Autodesk Inventor part; units mm, degrees
ref_plane "YZ Plane" through (0, 0, 0) normal (1, 0, 0) x (0, 1, 0)
ref_plane "XZ Plane" through (0, 0, 0) normal (0, 1, 0) x (-1, 0, 0)
ref_plane "XY Plane" through (0, 0, 0) normal (0, 0, 1) x (1, 0, 0)
sketch "Sketch1" plane through (0, 0, 0) normal (1, 0, 0) x (0, 1, 0)
  line L0 (0, 0) -> (3.175, 0)
  line L1 (3.175, -12.7) -> (0, -12.7)
  line L2 (0, -12.7) -> (0, 0)
  line L3 (3.175, 0) -> (28.575, 0)
  line L4 (3.175, -12.7) -> (28.575, -12.7)
  line L5 (12.065, -4.1275) -> (28.575, 0)
  line L6 (12.065, -8.5725) -> (28.575, -12.7)
  line L7 (12.065, -4.1275) -> (3.175, -4.1275)
  line L8 (12.065, -8.5725) -> (3.175, -8.5725)
  line L9 (3.175, -4.1275) -> (2.54, -4.1275)
  line L10 (2.54, -4.1275) -> (2.54, -8.5725)
  line L11 (2.54, -8.5725) -> (3.175, -8.5725)
  dimension "d0" = 3.175
  dimension "d1" = 12.7
  dimension "d2" = 25.4
  dimension "d3" = 0.635
extrude "Extrusion1" add sketch "Sketch1" along normal blind 88.9
sketch "Sketch2" plane through (0, 0, 0) normal (0, 0, 1) x (1, 0, 0)
  line L0 (70.7723, 45.5937) -> (70.7723, 36.3388)
  line L1 (0, 12.065) -> (88.9, 12.065)
  line L2 (70.7723, 36.3388) -> (70.7723, 45.5937)
  line L3 (70.7723, 45.5937) -> (88.9, 45.5937)
  line L4 (88.9, 45.5937) -> (70.7723, 45.5937)
  line L5 (70.7723, 45.5937) -> (79.5643, 35.1158)
  line L6 (88.9, 12.065) -> (88.9, 28.575)
  line L7 (88.9, 28.575) -> (57.2257, 28.575)
  line L8 (0, 28.575) -> (88.9, 28.575)
  line L9 (88.9, 0) -> (76.2, 0)
  line L10 (0, 0) -> (88.9, 0)
  line L11 (76.2, 0) -> (52.2227, 28.575)
  line L12 (52.2227, 28.575) -> (52.2227, 24.9497)
  line L13 (0, 28.575) -> (0, 0)
  line L14 (0, 0) -> (88.9, 0)
  line L15 (88.9, 28.575) -> (88.9, 0)
  line L16 (0, 28.575) -> (88.9, 28.575)
  dimension "d6" = 40
  dimension "d8" = 12.7
  dimension "d9" = 40
extrude "Extrusion2" add sketch "Sketch2" against normal blind 12.7 contours L11 L8 L7 L6 L1 | L1 L15 L9 L11
sketch "Sketch3" plane through (0, 0, 0) normal (0, 0, 1) x (1, 0, 0)
  line L0 (0, 28.575) -> (52.2227, 28.575)
  line L1 (52.2227, 28.575) -> (58.5727, 28.575)
  line L2 (52.2227, 28.575) -> (88.9, 28.575)
  line L3 (52.2227, 28.575) -> (66.0763, 12.065)
  line L4 (58.5727, 28.575) -> (89.629, -8.4365)
  line L5 (58.5727, 28.575) -> (106.8878, 28.575) construction
  line L6 (89.629, -8.4365) -> (99.364, 12.7806)
  line L7 (99.364, 12.7806) -> (87.0878, 39.7231)
  line L8 (87.0878, 39.7231) -> (61.7749, 33.0961)
  line L9 (61.7749, 33.0961) -> (58.5727, 28.575)
  point P0 (0, 0)
  dimension "d12" = 6.35
  dimension "d13" = 50
extrude "Extrusion3" cut sketch "Sketch3" against normal blind 12.7
properties part number "edge holder tip"
Geometry: final body of the model. Coordinates: model frame, mm. A direction names the side the tool comes from. Give positions to 0.01 mm unless a question says otherwise; leave off trailing zeros. Write each loop counter-clockwise with the first axis right and the second up, starting at its lowest first coordinate (ties: lowest second). Pieces come first, ordered by that corner, then holes.
(1) Cut plane B-B, the plane y = 23. Return loops of the section in (x, z), then the cut area to 3 significant figures.
(2) Mould query, pull axis Z, two halves, no side actions, for faces 1 (the flat face through (37, 7, -4.128)), 2 (the flat face through (37, 7, -8.572)), 3 (the flat face through (32, 14, 0)), 4 (the flat face through (0, 11, -3)). Classes: released by +Z, released by -Z, zero draft, split by the parting line, or undercut.
(3) Cut plane A-A, the plane x = 26.5. Return loops of the section in (y, z) (1 decimal), then the cut area to 3 significant figures.
(4) First-contact query: P1, Ø1, axis at y = 7, z = -4, coming from the +X side; P2, Ø1, axis at x = 72.5, y = 14, coming from the -Z side; P3, Ø4, axis at x = 47.5, z = -6.5, coming from the +Y side; P4, Ø4, axis at y = 24, z = -8.5, coming from the +X side. Flat tips, straight axial feed; report the tip coordinate or a pass-through.
(5) Ray query, line 1 (Z direction, x = 63, y = 3); line 2 (Y direction, x = 55.5, z = -6.75) (3 decimals); line 3 (Z direction, x = 57, y = 13.75). Return the intervals inside material, ascending.
(6) Access query for faces 5 (the flat face through (41, 0, -6)), 6 (the flat face through (60.87, 18.27, -6.26)). Directions: +Z, -Z, +X, -X, +Y, -Y. A direction counts if a zero-diameter tool reaches every point of the face in a straight line with its end or side. Return the directions, or none.
(7) Cut plane D-D, the plane z = -1.75. Return loops of the section in (x, y) (3 decimals).
(8) Cut plane C-C, the plane x = 64.5. Return loops of the section in (y, z) (1 decimal).
Values follow:
1. outline: (0, -12.7) - (63.25, -12.7) - (63.25, 0) - (0, 0) - (0, -1.39) - (56.9, -1.39) - (56.9, -11.31) - (0, -11.31) - close
1. area: 239 mm2
2. face 1: undercut
2. face 2: undercut
2. face 3: released by +Z
2. face 4: zero draft
3. outline: (0, -12.7) - (28.6, -12.7) - (12.1, -8.6) - (2.5, -8.6) - (2.5, -4.1) - (12.1, -4.1) - (28.6, 0) - (0, 0) - close
3. area: 179 mm2
4. P1: stops at x = 77.1
4. P2: passes through
4. P3: stops at y = 2.54
4. P4: stops at x = 64.09
5. line 1: z = -12.7 to -8.57, -4.13 to 0
5. line 2: y = 0 to 2.54, 24.669 to 28.575
5. line 3: z = -12.7 to -8.99, -3.71 to 0
6. face 5: +Z, -Z, +X, -X, -Y
6. face 6: -X
7. outline: (0, 0) - (82.55, 0) - (58.573, 28.575) - (52.223, 28.575) - (58.096, 21.575) - (0, 21.575) - close
8. outline: (0, -12.7) - (21.5, -12.7) - (21.5, 0) - (0, 0) - close; hole (2.5, -8.6) - (12.1, -8.6) - (13.9, -9) - (13.9, -3.7) - (12.1, -4.1) - (2.5, -4.1) - close
